```python
from build123d import *

# Parameters (mm, degrees)
SKICA1_W                 = 25
SKICA1_H                 = 70
SKICA1_R                 = 2.75
P_IDAT_VYSUNUT_M1_DEPTH  = 5
SKICA2_W                 = 25
SKICA2_H                 = 40
P_IDAT_VYSUNUT_M2_DEPTH  = 15
SKICA3_W                 = 6
SKICA3_H                 = 34
ODEBRAT_VYSUNUT_M1_DEPTH = 72.377271817
SKICA4_R                 = 4
ODEBRAT_VYSUNUT_M2_DEPTH = 2
SKICA5_R                 = 2.5
ODEBRAT_VYSUNUT_M3_DEPTH = 60.747879831


with BuildPart() as part:
    # Skica1 → Přidat vysunutím1 (new body)
    with BuildSketch(Plane(origin=(0, 0, 0), x_dir=(0, 0, -1), z_dir=(1, 0, 0))):
        with Locations((32.820037376, 16.388803686)):
            Rectangle(SKICA1_W, SKICA1_H)
        with Locations((26.320037376, 44.388803686)):
            Circle(SKICA1_R, mode=Mode.SUBTRACT)
        with Locations((39.320037376, 44.388803686)):
            Circle(SKICA1_R, mode=Mode.SUBTRACT)
        with Locations((26.320037376, -11.611196314)):
            Circle(SKICA1_R, mode=Mode.SUBTRACT)
        with Locations((39.320037376, -11.611196314)):
            Circle(SKICA1_R, mode=Mode.SUBTRACT)
    extrude(amount=P_IDAT_VYSUNUT_M1_DEPTH)

    # Skica2 → Přidat vysunutím2 (add)
    with BuildSketch(Plane(origin=(5, 0, 0), x_dir=(0, 0, -1), z_dir=(1, 0, 0))):
        with Locations((32.820037376, 16.388803686)):
            Rectangle(SKICA2_W, SKICA2_H)
    extrude(amount=P_IDAT_VYSUNUT_M2_DEPTH)

    # Skica3 → Odebrat vysunutím1 (cut, through all)
    with BuildSketch(Plane(origin=(20, 0, 0), x_dir=(0, 0, -1), z_dir=(1, 0, 0))):
        with Locations((26.320037376, 16.388803686)):
            Rectangle(SKICA3_W, SKICA3_H)
        with Locations((39.320037376, 16.388803686)):
            Rectangle(SKICA3_W, SKICA3_H)
    extrude(amount=-ODEBRAT_VYSUNUT_M1_DEPTH, mode=Mode.SUBTRACT)

    # Skica4 → Odebrat vysunutím2 (cut)
    with BuildSketch(Plane.XY.offset(-20.320037376)):
        with Locations((12.5, 16.388803686)):
            Circle(SKICA4_R)
    extrude(amount=-ODEBRAT_VYSUNUT_M2_DEPTH, mode=Mode.SUBTRACT)

    # Skica5 → Odebrat vysunutím3 (cut, through all)
    with BuildSketch(Plane.XY.offset(-22.320037376)):
        with Locations(Location((12.5, 16.388803686, 0), (0, 0, 90))):
            Circle(SKICA5_R)
    extrude(amount=-ODEBRAT_VYSUNUT_M3_DEPTH, mode=Mode.SUBTRACT)


solid = part.part
```
Could you check a few things on this model? Use its own coordinates, in mm. A direction names the side the tool comes from. Round coordinates to 2 decimals unless told otherwise and drop trailing zeros. Loops run counter-clockwise (first coordinate to the right, second up) from the corner with the lowest first, then second, coordinate; pieces in that order, holes last. Notation, with made-up numbers: M 69.5,7 L 86.5,7 A19 ccw 86.5,43 Z; hole C 7,2.5 d2. An arc over 180 degrees is marked long. Write item = value, one per line.
1. Will these pins go through, and if not, where does the flat tip stop? P1, Ø4, axis at x = 11, y = 16.5, coming from the +Z side; P2, Ø7.5, axis at x = 14.5, z = -31, coming from the +Y side; P3, Ø3.5, axis at y = -11.61, z = -26.32, coming from the -X side; P4, Ø3, axis at y = 41, z = -38, coming from the +X side.
Results below:
P1 = -22.32
P2 = 36.39
P3 = through
P4 = 5
2. I want a section at B-B, the plane z = -32. Write out the boundary of the cut face in (x, y), and give its area (3 significant figures).
Results below:
outline = M 0,-18.61 L 5,-18.61 L 5,-3.61 L 20,-3.61 L 20,36.39 L 5,36.39 L 5,51.39 L 0,51.39 Z; hole C 12.5,16.39 d5
area = 930 mm²
3. I want a section at D-D, the plane z = -38. Write out the boundary of the cut face in (x, y).
Results below:
outline = M 0,-18.61 L 5,-18.61 L 5,-14.02 L 0,-14.02 Z; M 0,-9.2 L 5,-9.2 L 5,-3.61 L 20,-3.61 L 20,-0.61 L 0,-0.61 Z; M 0,33.39 L 20,33.39 L 20,36.39 L 5,36.39 L 5,41.98 L 0,41.98 Z; M 0,46.8 L 5,46.8 L 5,51.39 L 0,51.39 Z
4. I need wall thicknesses on probe 1 along Z at (x, y) = (8.5, 30); probe 2 along Y at (x, z) = (8.5, -39.5); probe 3 along Y at (x, z) = (2, -40). Which ranges of each line are inside material? Lowest first, please.
Results below:
probe_1 = -45.32 to -42.32, -36.32 to -29.32, -23.32 to -20.32
probe_2 = -3.61 to -0.61, 33.39 to 36.39
probe_3 = -18.61 to -14.28, -8.95 to -0.61, 33.39 to 41.72, 47.05 to 51.39
5. I want a section at A-A, the plane x = 12.5. Write out the boundary of the cut face in (y, z), and give its area (3 significant figures).
Results below:
outline = M -3.61,-45.32 L 13.89,-45.32 L 13.89,-42.32 L -0.61,-42.32 L -0.61,-36.32 L 13.89,-36.32 L 13.89,-29.32 L -0.61,-29.32 L -0.61,-23.32 L 13.89,-23.32 L 13.89,-22.32 L 12.39,-22.32 L 12.39,-20.32 L -3.61,-20.32 Z; M 18.89,-45.32 L 36.39,-45.32 L 36.39,-20.32 L 20.39,-20.32 L 20.39,-22.32 L 18.89,-22.32 L 18.89,-23.32 L 33.39,-23.32 L 33.39,-29.32 L 18.89,-29.32 L 18.89,-36.32 L 33.39,-36.32 L 33.39,-42.32 L 18.89,-42.32 Z
area = 521 mm²
6. Which directions (+Z, -Z, +X, -X, +Y, -Y) give clear straight access to the entire face, cutting with the end or side of a thin tool? Please do faces 1 (the face through (12, -3.611, -33)), 2 (the face through (8, 16, -42.32)), 3 (the face through (11.979, 20.355, -21.306)), 4 (the face through (5, 44, -33)), 5 (the face through (14.72, 17.54, -32.77)).
Results below:
face_1 = +Z, -Z, +X, -Y
face_2 = +X, -X
face_3 = +Z
face_4 = +Z, -Z, +X, +Y
face_5 = +Z, -Z
7. I want a section at C-C, the plane x = 7. Write out the boundary of the cut face in (y, z), and give its area (3 significant figures).
Results below:
outline = M -3.61,-45.32 L 36.39,-45.32 L 36.39,-20.32 L -3.61,-20.32 Z; hole M -0.61,-42.32 L 33.39,-42.32 L 33.39,-36.32 L -0.61,-36.32 Z; hole M -0.61,-29.32 L 33.39,-29.32 L 33.39,-23.32 L -0.61,-23.32 Z
area = 592 mm²
8. Thinking about a two-plate mould opening in Y: for faces 6 (the face through (2, 51.389, -33)), 7 (the face through (14.72, 17.54, -43.8)), 8 (the face through (5, -11, -33)), which applies, +Y half, -Y half, draft (parallel to the pull), parting line (faces both ways), or undercut?
Results below:
face_6 = +Y half
face_7 = undercut
face_8 = draft
